The model under review builds one solid part; all positions refer to its coordinate system, in mm. A direction names the side the tool comes from. Round coordinates to 2 decimals unless told otherwise and drop trailing zeros. Order: outer loops, then holes, each group sorted by start corner. A loop starts at its lowest first (then second) coordinate and runs counter-clockwise, first axis right, second up.
1) Consider section C-C (y = -17). Give the boundary of the cut face in (x, z) (3 decimals), then the cut area to 3 significant figures.
2) Consider section B-B (y = -30). Give the boundary of the cut face in (x, z) (3 decimals).
3) Consider section A-A (z = -2.5). Give the boundary of the cut face in (x, y) (3 decimals), then the cut area to 3 significant figures.
4) To check wall thickness, follow L1, parallel to Y at x = 40, z = 48; L2, parallel to Z at x = -6, y = 25.5 (3 decimals); L3, parallel to Z at x = 66, y = 1 (3 decimals). State the ranges of each line that lie inside material, in increasing order.
5) Clearance check with flat-ended pins moving along their axes: P1, Ø5, axis at y = -13, z = 15.5, coming from the -X side (3 decimals); P2, Ø1.5, axis at x = 16, z = 56, coming from the +Y side; P3, Ø23, axis at x = 72, y = 6, coming from the -Z side. State where each tip first meets the part, or that it passes through.
6) Machinability: for faces 1 (the face through (22.225, -17, 18)), 2 (the face through (41.275, -1, 4)), 3 (the face through (60, 0, 61.925)), which of the approach directions +Z, -Z, +X, -X, +Y, -Y give a long, thin tool a straight path to every point of the face, cutting with its end or side? Answer none if there is none.
7) Mouldability with a two-part tool opening along Z and no side actions: class faces 4 (the face through (-39.365, 61.689, -0.133)), 5 (the face through (-1, -1, -9.525)), 6 (the face through (85, 0, 66.675)) as pulls with the +Z half, pulls with the -Z half, needs draft (parallel to the pull), parting line crosses it, or undercut.
from build123d import *

# Parameters (mm, degrees)
F1_DEPTH = 63.5
F0_W     = 25.4749524852
F0_H     = 19.05
F2_DEPTH = 25.4
F3_DEPTH = 7.9375
F5_R     = 6.35


with BuildPart() as f1:
    # F0 (on Front) → F1 (new body, symmetric)
    with BuildSketch(Plane.XZ):
        Polygon((41.275, -9.525), (41.275, 9.525), (22.225, 9.525), (-41.275, 9.525), (-41.275, -9.525), align=None)
    extrude(amount=F1_DEPTH, both=True)

    # F0 (on Front) → F2 (join, symmetric)
    with BuildSketch(Plane.XZ):
        with BuildLine():
            Line((22.225, 9.525), (41.275, 9.525))
            Line((41.275, 9.525), (41.275, 27.0002))
            ThreePointArc((41.275, 27.0002), (45.9246798487, 38.2255201513), (57.15, 42.8752))
            Line((57.15, 42.8752), (60.325, 42.8752))
            Line((60.325, 42.8752), (60.325, 61.9252))
            Line((60.325, 61.9252), (57.15, 61.9252))
            ThreePointArc((57.15, 61.9252), (53.0680704253, 61.6858378916), (49.0420927056, 60.9710325524))
            ThreePointArc((49.0420927056, 60.9710325524), (29.7371901544, 48.6402896803), (22.225, 27.0002))
            Line((22.225, 27.0002), (22.225, 9.525))
        make_face()
        with Locations((73.0624762426, 52.4002)):
            Rectangle(F0_W, F0_H)
    extrude(amount=F2_DEPTH, both=True)

    # F0 (on Front) → F3 (join, symmetric)
    with BuildSketch(Plane.XZ):
        with BuildLine():
            Line((-41.275, 9.525), (22.225, 9.525))
            Line((22.225, 9.525), (22.225, 27.0002))
            ThreePointArc((22.225, 27.0002), (29.7371901544, 48.6402896803), (49.0420927056, 60.9710325524))
            add(Edge.make_bspline(
                [(-41.275, 9.525), (-41.1753505468, 41.8217629194), (0, 59.1593452108), (49.0420927056, 60.9710325524)],
                knots=[0, 0, 0, 0, 103.941673549, 103.941673549, 103.941673549, 103.941673549], degree=3))
        make_face()
    extrude(amount=F3_DEPTH, both=True)

    # F0 (on Front) → F4 (revolve)
    with BuildSketch(Plane.XZ):
        Polygon((85.7999524852, 61.9252), (85.7999524852, 42.8752), (85.7999524852, 38.1), (111.125, 38.1), (111.125, 66.675), (85.7999524852, 66.675), align=None)
    revolve(axis=Axis((85.7999524852, 0, 52.3875), (0, 0, 1)))

    # F5
    f5_edges = [f1.edges().sort_by_distance(p)[0] for p in [
        (41.275, -63.5, 0),
        (41.275, 63.5, 0),
        (-41.275, 63.5, 0),
        (-41.275, -63.5, 0),
    ]]
    fillet(f5_edges, radius=F5_R)


solid = f1.part
Answer below:
1. outline: (-41.275, -9.525) - (41.275, -9.525) - (41.275, 27) arc R15.875 cw to (57.15, 42.875) - (67.029, 42.875) - (67.029, 38.1) - (104.571, 38.1) - (104.571, 66.675) - (67.029, 66.675) - (67.029, 61.925) - (57.15, 61.925) arc R34.925 ccw to (22.225, 27) - (22.225, 9.525) - (-41.275, 9.525) - close
1. area: 3,930 mm2
2. outline: (-41.275, -9.525) - (41.275, -9.525) - (41.275, 9.525) - (-41.275, 9.525) - close
3. outline: (-41.275, -57.15) arc R6.35 ccw to (-34.925, -63.5) - (34.925, -63.5) arc R6.35 ccw to (41.275, -57.15) - (41.275, 57.15) arc R6.35 ccw to (34.925, 63.5) - (-34.925, 63.5) arc R6.35 ccw to (-41.275, 57.15) - close
3. area: 10,400 mm2
4. L1: y = -25.4 to 25.4
4. L2: z = -9.525 to 9.525
4. L3: z = 38.1 to 66.675
5. P1: stops at x = 22.225
5. P2: stops at y = 7.94
5. P3: stops at z = 38.1
6. face 1: +Z, -X, -Y
6. face 2: -Z, +X, +Y, -Y
6. face 3: +Z, -X
7. face 4: needs draft
7. face 5: pulls with the -Z half
7. face 6: pulls with the +Z half
